```python
from build123d import *

# Parameters (mm, degrees)
F2_DEPTH = 41.275
F3_DEPTH = 41.275
F4_W     = 5.590443
F4_H     = 1.984375
F4_H_2   = 3.175
F5_DEPTH = 4.7625
F7_DEPTH = 2.38125
F8_DEPTH = 2.38125


with BuildPart() as f2:
    # F1 (on Top) → F2 (new body)
    with BuildSketch(Plane.XY):
        with BuildLine():
            ThreePointArc((8.334375, -11.1125), (12.424153, -6.212076), (13.890625, 0))
            ThreePointArc((13.890625, 0), (12.424153, 6.212076), (8.334375, 11.1125))
            ThreePointArc((8.334375, 11.1125), (-7.53772, 11.667572), (-13.556196, -3.029687))
            ThreePointArc((-13.556196, -3.029687), (-11.667572, -7.53772), (-8.334375, -11.1125))
            ThreePointArc((-8.334375, -11.1125), (0, -13.890625), (8.334375, -11.1125))
        make_face()
        with BuildLine():
            ThreePointArc((7.451328, -2.735254), (-7.9375, 0), (7.451328, 2.735254))
            ThreePointArc((7.451328, 2.735254), (9.721783, 2.129392), (10.715625, 0))
            ThreePointArc((10.715625, 0), (9.721783, -2.129392), (7.451328, -2.735254))
        make_face(mode=Mode.SUBTRACT)
        with BuildLine():
            ThreePointArc((7.451328, 2.735254), (7.815012, 1.389063), (7.9375, 0))
            ThreePointArc((7.9375, 0), (7.815012, -1.389063), (7.451328, -2.735254))
            ThreePointArc((7.451328, -2.735254), (9.721783, -2.129392), (10.715625, 0))
            ThreePointArc((10.715625, 0), (9.721783, 2.129392), (7.451328, 2.735254))
        make_face()
    extrude(amount=F2_DEPTH)

    # F0 (on Top) → F3 (join)
    with BuildSketch(Plane.XY):
        with BuildLine():
            ThreePointArc((7.879068, 11.439832), (12.296232, 6.46159), (13.890625, 0))
            ThreePointArc((13.890625, 0), (12.540847, -5.972991), (8.753834, -10.785168))
            Line((8.753834, -10.785168), (15.875, -10.785168))
            Line((15.875, -10.785168), (15.875, 0.327332))
            Line((15.875, 0.327332), (15.875, 11.439832))
            Line((15.875, 11.439832), (7.879068, 11.439832))
        make_face()
    extrude(amount=F3_DEPTH)

    # F4 (on face) → F5 (cut)
    with BuildSketch(Plane.YZ.offset(15.875)):
        with Locations((0.327332, 25.201562)):
            Rectangle(F4_W, F4_H)
        with Locations((0.327332, 20.6375)):
            Rectangle(F4_W, F4_H_2)
        with Locations((0.327332, 16.073438)):
            Rectangle(F4_W, F4_H)
    extrude(amount=-F5_DEPTH, mode=Mode.SUBTRACT)

    # F6 (on face) → F7 (cut)
    with BuildSketch(Plane.XY.offset(41.275)):
        with BuildLine():
            ThreePointArc((7.451328, -2.735254), (9.721783, -2.129392), (10.715625, 0))
            ThreePointArc((10.715625, 0), (9.721783, 2.129392), (7.451328, 2.735254))
            ThreePointArc((7.451328, 2.735254), (7.815012, 1.389062), (7.9375, 0))
            ThreePointArc((7.9375, 0), (7.815012, -1.389063), (7.451328, -2.735254))
        make_face()
    extrude(amount=-F7_DEPTH, mode=Mode.SUBTRACT)

    # F1 (on Top) → F8 (cut)
    with BuildSketch(Plane.XY):
        with BuildLine():
            ThreePointArc((7.451328, 2.735254), (7.815012, 1.389063), (7.9375, 0))
            ThreePointArc((7.9375, 0), (7.815012, -1.389063), (7.451328, -2.735254))
            ThreePointArc((7.451328, -2.735254), (9.721783, -2.129392), (10.715625, 0))
            ThreePointArc((10.715625, 0), (9.721783, 2.129392), (7.451328, 2.735254))
        make_face()
    extrude(amount=F8_DEPTH, mode=Mode.SUBTRACT)


solid = f2.part
```
Design review of the part built by this model. Coordinates are the model's own, in mm. A direction names the side the tool comes from. Round coordinates to 2 decimals unless told otherwise and drop trailing zeros. Write each loop counter-clockwise with the first axis right and the second up, starting at its lowest first coordinate (ties: lowest second). Pieces come first, ordered by that corner, then holes.
Item 1: We need section C-C on z = 27.5. Write out the cut boundary in (x, y) (1 decimal), and give its area (3 significant figures).
Item 2: For faces 1 (the flat face through (12, -10.785, 20)), 2 (the flat face through (7.4, 3.3, 0)), 3 (the flat face through (14, -2.468, 21)), 4 (the flat face through (12, 11.44, 20)), list the 3-axis set-ups (+Z, -Z, +X, -X, +Y, -Y) from which the entire face can be reached by the end or side of a thin tool; tool diameter is ignored.
Item 3: The part is to be moulded in two halves that separate along Z. For faces 5 (the flat face through (14, 0, 24.209)), 6 (the flat face through (9, 0, 2.381)), 7 (the flat face through (9, 0, 38.894)), 8 (the cylindrical face through (-7.93, -0.31, 20.35)), say which applies: +Z half, -Z half, draft (parallel to the pull), parting line (faces both ways), or undercut.
Item 4: Clearance check with flat-ended pins moving along their axes: pin 1 Ø6.5 at (x, z) = (12.5, 22) entering from +Y; pin 2 Ø1.6 at (x, y) = (9.5, -1) entering from -Z; pin 3 Ø1 at (x, z) = (13, 21) entering from -Y; pin 4 Ø14.5 at (x, y) = (0, 0) entering from -Z. State where each tip first meets the part, or that it passes through.
Item 5: We need section A-A on x = 0. Write out the cut boundary in (y, z) (1 decimal).
Item 6: We need section D-D on x = 12. Write out the cut boundary in (y, z) (3 decimals).
Item 7: For probe 1 along Z at (x, y) = (13, -1.5) (3 decimals); probe 2 along Y at (x, z) = (0, 12); probe 3 along Y at (x, z) = (4.75, 23.5), list the stretches that pass through material, from the lowest coordinate up.
Returned:
1. outline: (7.9, 11.4) arc R13.9 ccw (long way) to (8.8, -10.8) - (15.9, -10.8) - (15.9, 11.4) - close; hole (7.5, -2.7) arc R7.9 ccw to (7.9, 0) arc R7.9 ccw to (7.5, 2.7) arc R7.9 ccw (long way) to start
1. area: 490 mm2
2. face 1: +Z, -Z, +X, -Y
2. face 2: -Z, +X, -X, +Y, -Y
2. face 3: +X
2. face 4: +Z, -Z, +X, +Y
3. face 5: undercut
3. face 6: -Z half
3. face 7: +Z half
3. face 8: draft
4. pin 1: stops at y = 11.44
4. pin 2: stops at z = 2.38
4. pin 3: stops at y = -10.79
4. pin 4: passes through
5. outline: (-13.9, 0) - (-7.9, 0) - (-7.9, 41.3) - (-13.9, 41.3) - close; (7.9, 0) - (13.9, 0) - (13.9, 41.3) - (7.9, 41.3) - close
6. outline: (-10.785, 0) - (11.44, 0) - (11.44, 41.275) - (-10.785, 41.275) - close; hole (-2.468, 15.081) - (3.123, 15.081) - (3.123, 17.066) - (-2.468, 17.066) - close; hole (-2.468, 19.05) - (3.123, 19.05) - (3.123, 22.225) - (-2.468, 22.225) - close; hole (-2.468, 24.209) - (3.123, 24.209) - (3.123, 26.194) - (-2.468, 26.194) - close
7. probe 1: z = 0 to 15.081, 17.066 to 19.05, 22.225 to 24.209, 26.194 to 41.275
7. probe 2: y = -13.89 to -7.94, 7.94 to 13.89
7. probe 3: y = -13.05 to -6.36, 6.36 to 13.05
